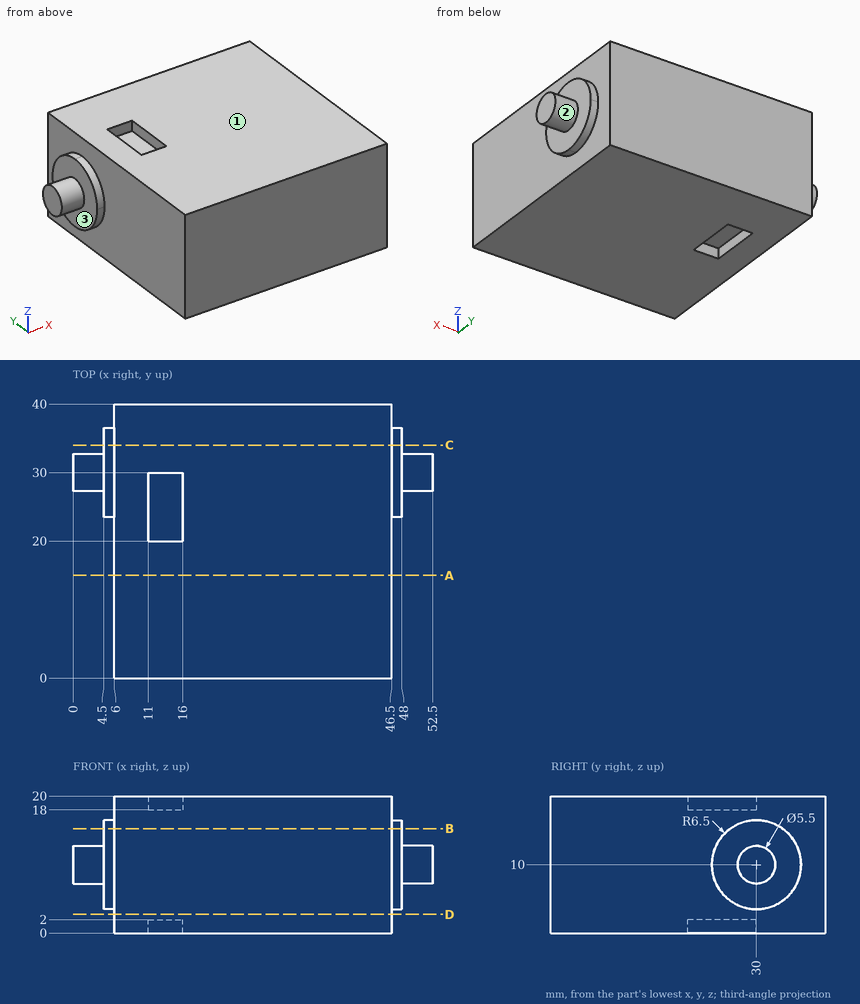
Drawing for the job (mm, zero at the part's lowest x, y, z). A direction names the side the tool comes from. Round coordinates to 2 decimals unless told otherwise and drop trailing zeros. Write each loop counter-clockwise with the first axis right and the second up, starting at its lowest first coordinate (ties: lowest second). Pieces come first, ordered by that corner, then holes. Notation, with made-up numbers: M 71,22.5 L 92,22.5 A22 ccw 92,39.5 Z; hole C 32.5,-7 d10. An arc over 180 degrees is marked long. Answer as a JSON object with one key per item and string values. Group by question number.
(1) Cut at C-C (y = 34). Give the cut face in (x, z), and give its area (3 significant figures).
(2) Flat gauge pins, fed straight in: pin 1 (2.5 mm diameter, centred on x = 13.5, y = 22.5, fed in from -Z); pin 2 (10 mm diameter, centred on x = 13.5, y = 21.5, fed in from +Z); pin 3 (10 mm diameter, centred on y = 21, z = 7.5, fed in from +X); pin 4 (1.6 mm diameter, centred on y = 23, z = 1, fed in from +X). Where does each tip first touch, or does it go through?
(3) Drill centre lines: L1, parallel to X at y = 21, z = 1.25; L2, parallel to X at y = 6, z = 1.5; L3, parallel to Z at x = 15, y = 21. Where is each one in solid material? Low to high.
(4) Cut at B-B (z = 15.25). Give the cut face in (x, y).
(5) Which spindle directions (+Z, -Z, +X, -X, +Y, -Y) get a long thin tool onto all of the face, cutting with end or side? Do the marked faces 1, 2 and 3. Say none if no direction does.
(6) Cut at A-A (y = 15). Give the cut face in (x, z), and give its area (3 significant figures).
(7) Cut at D-D (z = 2.75). Give the cut face in (x, y).
Responses:
{
 "1": {"outline": "M 4.5,4.88 L 6,4.88 L 6,0 L 46.5,0 L 46.5,4.88 L 48,4.88 L 48,15.12 L 46.5,15.12 L 46.5,20 L 6,20 L 6,15.12 L 4.5,15.12 Z", "area": "841 mm2"},
 "2": {"pin 1": "stops at z = 2", "pin 2": "stops at z = 20", "pin 3": "stops at x = 48", "pin 4": "stops at x = 46.5"},
 "3": {"L1": "x = 6 to 11, 16 to 46.5", "L2": "x = 6 to 46.5", "L3": "z = 2 to 18"},
 "4": {"outline": "M 4.5,26.17 L 6,26.17 L 6,0 L 46.5,0 L 46.5,26.17 L 48,26.17 L 48,33.83 L 46.5,33.83 L 46.5,40 L 6,40 L 6,33.83 L 4.5,33.83 Z"},
 "5": {"face 1": "+Z, +X, -X, +Y, -Y", "face 2": "+X", "face 3": "-X"},
 "6": {"outline": "M 6,0 L 46.5,0 L 46.5,20 L 6,20 Z", "area": "810 mm2"},
 "7": {"outline": "M 6,0 L 46.5,0 L 46.5,40 L 6,40 Z"}
}
